```python
from build123d import *

# Parameters (mm, degrees)
SKETCH1_W           = 340
SKETCH1_H           = 254
BOSS_EXTRUDE1_DEPTH = 5
CUT_EXTRUDE1_REACH  = 12
SKETCH2_W           = 254
SKETCH2_H           = 196.85


with BuildPart() as part:
    # Sketch1 → Boss-Extrude1 (new body, symmetric)
    with BuildSketch(Plane(origin=(0, 0, 0), x_dir=(1, 0, 0), z_dir=(0, 1, 0))):
        Rectangle(SKETCH1_W, SKETCH1_H)
    extrude(amount=BOSS_EXTRUDE1_DEPTH, both=True)

    # Sketch2 → Cut-Extrude1 (cut, up to next)
    with BuildSketch(Plane(origin=(0, 5, 0), x_dir=(1, 0, 0), z_dir=(0, 1, 0)), mode=Mode.PRIVATE) as cut_extrude1_sk1:
        Rectangle(SKETCH2_W, SKETCH2_H)
    cut_extrude1_tool1 = extrude(cut_extrude1_sk1.sketch, amount=-CUT_EXTRUDE1_REACH, mode=Mode.PRIVATE) & part.part
    add(cut_extrude1_tool1.solids().sort_by_distance((0, 5, 0))[0], mode=Mode.SUBTRACT)


solid = part.part
```
The model under review builds one solid part; all positions refer to its coordinate system, in mm. A direction names the side the tool comes from. Give positions to 0.01 mm unless a question says otherwise; leave off trailing zeros. Write each loop counter-clockwise with the first axis right and the second up, starting at its lowest first coordinate (ties: lowest second). Pieces come first, ordered by that corner, then holes. Notation, with made-up numbers: M -30.75,17 L 18.25,17 A19 ccw 18.25,51 Z; hole C 28,13.5 d11. An arc over 180 degrees is marked long. Write each question's results on one line, items separated by ' | '. Start each with the question number.
1. Mouldability with a two-part tool opening along X and no side actions: class faces 1 (the flat face through (-170, 0, 2)), 2 (the flat face through (-2, 5, 111)), 3 (the flat face through (-2, 0, 98.425)) as released by +X, released by -X, zero draft, split by the parting line, or undercut.
2. We need section B-B (x = -83). Write out the cut boundary in (y, z) (3 decimals).
3. For faces 4 (the flat face through (127, 0, 1)), 5 (the flat face through (-2, -5, 111)), list the 3-axis set-ups (+Z, -Z, +X, -X, +Y, -Y) from which the entire face can be reached by the end or side of a thin tool; tool diameter is ignored.
4. We need section A-A (z = -5). Write out the cut boundary in (x, y), and give its area (3 significant figures).
5. For probe 1 along Z at (x, y) = (-30, -3) (3 decimals); probe 2 along X at (y, z) = (-0.5, 3.5), list the stretches that pass through material, from the lowest coordinate up. Write a range as [from, to].
6. We need section C-C (y = 3.5). Write out the cut boundary in (x, z) (3 decimals).
Results found:
1) face 1: released by -X | face 2: zero draft | face 3: undercut
2) outline: M -5,-127 L 5,-127 L 5,-98.425 L -5,-98.425 Z; M -5,98.425 L 5,98.425 L 5,127 L -5,127 Z
3) face 4: +Y, -Y | face 5: +Z, -Z, +X, -X, -Y
4) outline: M -170,-5 L -127,-5 L -127,5 L -170,5 Z; M 127,-5 L 170,-5 L 170,5 L 127,5 Z | area: 860 mm^2
5) probe 1: z = [-127, -98.425], [98.425, 127] | probe 2: x = [-170, -127], [127, 170]
6) outline: M -170,-127 L 170,-127 L 170,127 L -170,127 Z; hole M -127,-98.425 L 127,-98.425 L 127,98.425 L -127,98.425 Z
